Build history of the part. All positions in model axes, mm. Face numbers are marked on the shaded views. A direction names the side the tool comes from. Round coordinates to 2 decimals unless told otherwise and drop trailing zeros. Loops run counter-clockwise (first coordinate to the right, second up) from the corner with the lowest first, then second, coordinate; pieces in that order, holes last. Notation, with made-up numbers: (-38.75, 1) -> (11.25, 1) arc R9 cw to (11.25, 12) -> close; hole circle Ø3 at (18.5, 45). An arc over 180 degrees is marked (long way). Put each result on its own line as item: value. Start each with the question number.
Item 1: Cut at A-A, the plane y = -15. List the corners of the cut face in (x, z).
Item 2: Cut at C-C, the plane z = 10.5. List the corners of the cut face in (x, y).
Item 3: Tool access for the marked faces 1, 2 and 3: list every direction of +Z, -Z, +X, -X, +Y, -Y with a clear straight run to the whole face (end or side of a thin tool).
Item 4: Drill centre lines: probe 1 along Z at (x, y) = (20, -25.5); probe 2 along Z at (x, y) = (43, -24.25); probe 3 along Y at (x, z) = (0, 11.75). Where is each one in solid material? Low to high. Write a range as [from, to].
Item 5: Cut at B-B, the plane x = 63. List the corners of the cut face in (y, z).
Item 6: Pull direction Y, two halves, no side cores. Call the marked faces 4, 5, 6 and 7: +Y half, -Y half, draft (parallel to the pull), parting line (faces both ways), or undercut.
Item 7: Cut at D-D, the plane y = -24.5. List the corners of the cut face in (x, z), plus the area to 3 significant figures.
Item 8: Flat gauge pins, fed straight in: pin 1 Ø9 at (x, y) = (57, -13) entering from +Z; pin 2 Ø4 at (y, z) = (-12.5, 6) entering from -X; pin 3 Ø6 at (x, y) = (33, -17) entering from -Z. Where does each tip first touch, or does it go through?
```python
from build123d import *

# Parameters (mm, degrees)
PAD_DEPTH       = 30
PAD001_DEPTH    = 7
PAD002_DEPTH    = 7
SKETCH004_R     = 8
POCKET_DEPTH    = 21.244539
SKETCH006_R     = 8
POCKET001_DEPTH = 21.244539


with BuildPart() as part:
    # Sketch → Pad (new body)
    with BuildSketch(Plane.XZ):
        Polygon((0, 14.243539), (27, 14.243539), (41.04, 0), (68.04, 0), (68.04, -7), (41.04, -7), (27, 7.243539), (0, 7.243539), align=None)
    extrude(amount=PAD_DEPTH)

    # Sketch002 (on DatumPlane) → Pad001 (join)
    with BuildSketch(Plane(origin=(0, -15, 14.243539), x_dir=(1, 0, 0), z_dir=(0, 0, 1))):
        with BuildLine():
            ThreePointArc((0, 15), (-15, 0), (0, -15))
            Line((0, 15), (0, -15))
        make_face()
    extrude(amount=-PAD001_DEPTH)

    # Sketch003 (on DatumPlane) → Pad002 (join)
    with BuildSketch(Plane(origin=(68.04, -15, -7), x_dir=(1, 0, 0), z_dir=(0, 0, 1))):
        with BuildLine():
            ThreePointArc((0, -15), (14.999969, 0), (0, 15))
            Line((0, 15), (0, -15))
        make_face()
    extrude(amount=PAD002_DEPTH)

    # Sketch004 → Pocket (cut, through all)
    with BuildSketch(Plane(origin=(68.039969, -15, -7), x_dir=(0, -1, 0), z_dir=(0, 0, -1))):
        Circle(SKETCH004_R)
    extrude(amount=-POCKET_DEPTH, mode=Mode.SUBTRACT)

    # Sketch006 (on DatumPlane) → Pocket001 (cut, through all)
    with BuildSketch(Plane(origin=(0, -15, 14.243539), x_dir=(1, 0, 0), z_dir=(0, 0, 1))):
        Circle(SKETCH006_R)
    extrude(amount=-POCKET001_DEPTH, mode=Mode.SUBTRACT)


solid = part.part
```
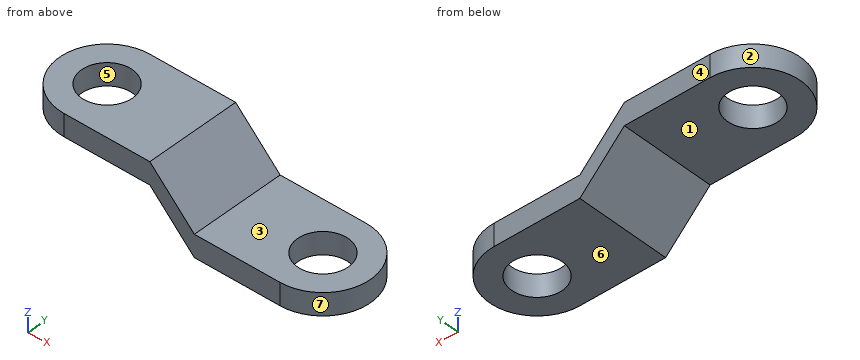
Reply:
1. outline: (-15, 7.24) -> (-8, 7.24) -> (-8, 14.24) -> (-15, 14.24) -> close; (8, 7.24) -> (27, 7.24) -> (41.04, -7) -> (60.04, -7) -> (60.04, 0) -> (41.04, 0) -> (27, 14.24) -> (8, 14.24) -> close; (76.04, -7) -> (83.04, -7) -> (83.04, 0) -> (76.04, 0) -> close
2. outline: (0, -30) -> (30.69, -30) -> (30.69, 0) -> (0, 0) arc R15 ccw to start; hole circle Ø16 at (0, -15)
3. face 1: -Z, -X, +Y, -Y
3. face 2: +Z, -Z, -X
3. face 3: +Z, +X, +Y, -Y
4. probe 1: z = [7.24, 14.24]
4. probe 2: z = [-7, 0]
4. probe 3: y = [-30, -23], [-7, 0]
5. outline: (-30, -7) -> (-21.21, -7) -> (-21.21, 0) -> (-30, 0) -> close; (-8.79, -7) -> (0, -7) -> (0, 0) -> (-8.79, 0) -> close
6. face 4: +Y half
6. face 5: undercut
6. face 6: draft
6. face 7: parting line
7. outline: (-11.61, 7.24) -> (27, 7.24) -> (41.04, -7) -> (79.65, -7) -> (79.65, 0) -> (41.04, 0) -> (27, 14.24) -> (-11.61, 14.24) -> close
7. area: 639 mm^2
8. pin 1: stops at z = 0
8. pin 2: stops at x = -14.97
8. pin 3: stops at z = -1.89
